Source: CAD feature listing. Evaluate the final solid. Frame: model axes, mm. A direction names the side the tool comes from. Coordinates: 2 decimals unless noted, no trailing zeros. Order: outer loops, then holes, each group sorted by start corner. A loop starts at its lowest first (then second) coordinate and runs counter-clockwise, first axis right, second up. Notation, with made-up numbers: (57, 57.25) - (97, 57.25) arc R24 cw to (97, 78.25) - close; hole circle Ø4 at (74.25, 22.25). An arc over 180 degrees is marked (long way). One line per question, with ' | ' between items.
from build123d import *

# Parameters (mm, degrees)
SKETCH1_R           = 60
BOSS_EXTRUDE1_DEPTH = 40
SKETCH2_R           = 30
BOSS_EXTRUDE2_DEPTH = 355
SKETCH3_W           = 35
SKETCH3_H           = 68.96676223
CUT_EXTRUDE1_DEPTH  = 45
SKETCH4_R           = 5
BOSS_EXTRUDE3_DEPTH = 35


with BuildPart() as part:
    # Sketch1 → Boss-Extrude1 (new body)
    with BuildSketch(Plane(origin=(0, 0, 0), x_dir=(0, 0, -1), z_dir=(1, 0, 0))):
        Circle(SKETCH1_R)
    extrude(amount=BOSS_EXTRUDE1_DEPTH)

    # Sketch2 → Boss-Extrude2 (add)
    with BuildSketch(Plane(origin=(40, 0, 0), x_dir=(0, 0, -1), z_dir=(1, 0, 0))):
        Circle(SKETCH2_R)
    extrude(amount=BOSS_EXTRUDE2_DEPTH)

    # Sketch3 → Cut-Extrude1 (cut)
    with BuildSketch(Plane(origin=(395, 0, 0), x_dir=(0, 0, -1), z_dir=(1, 0, 0))):
        Rectangle(SKETCH3_W, SKETCH3_H)
    extrude(amount=-CUT_EXTRUDE1_DEPTH, mode=Mode.SUBTRACT)

    # Sketch4 → Boss-Extrude3 (add)
    with BuildSketch(Plane.XY.offset(-17.5)):
        with Locations(Location((385, 0, 0), (0, 0, 180))):
            Circle(SKETCH4_R)
    extrude(amount=BOSS_EXTRUDE3_DEPTH)


solid = part.part
(1) Cut plane B-B (z = 0). Return the cut outline in (x, y), and give its area (3 significant figures).
Taken from the geometry:
outline: (0, -60) - (40, -60) - (40, -30) - (350, -30) - (350, 30) - (40, 30) - (40, 60) - (0, 60) - close; circle Ø10 at (385, 0) | area: 23,500 mm²
(2) Pin query (flat end, axial travel): P1, Ø12, axis at x = 104, z = 38, coming from the +Y side; P2, Ø13.5, axis at x = 369, y = 0.5, coming from the -Z side; P3, Ø5, axis at x = 327, y = 11.5, coming from the +Z side; P4, Ø6, axis at x = 115.5, z = 14, coming from the -Y side. Return the tip coordinate at first contact, or that it passes through.
Taken from the geometry:
P1: passes through | P2: stops at z = -30 | P3: stops at z = 28.62 | P4: stops at y = -27.91
(3) Material intervals for L1, parallel to X at y = -46.5, z = 34; L2, parallel to Y at x = 208.5, z = -2; L3, parallel to Z at x = 109, y = 13, sorted ascending. Write a range as from..to.
Taken from the geometry:
L1: x = 0..40 | L2: y = -29.93..29.93 | L3: z = -27.04..27.04
(4) Pull-direction query (Z, two-part tool) for faces 3 (the cylindrical face through (215.02, 1.32, 29.97)), 4 (the cylindrical face through (380.23, -1.5, -0.25)), 5 (the flat face through (395, 0, -22)); classes: pulls with the +Z half, pulls with the -Z half, needs draft (parallel to the pull), parting line crosses it, or undercut.
Taken from the geometry:
face 3: parting line crosses it | face 4: undercut | face 5: needs draft
(5) Cut plane D-D (z = -48). Return the cut outline in (x, y), and give its area (3 significant figures).
Taken from the geometry:
outline: (0, -36) - (40, -36) - (40, 36) - (0, 36) - close | area: 2,880 mm²
(6) Cut plane A-A (y = 0). Return the cut outline in (x, z).
Taken from the geometry:
outline: (0, -60) - (40, -60) - (40, -30) - (395, -30) - (395, -17.5) - (390, -17.5) - (390, 17.5) - (395, 17.5) - (395, 30) - (40, 30) - (40, 60) - (0, 60) - close; hole (350, -17.5) - (380, -17.5) - (380, 17.5) - (350, 17.5) - close
(7) Set-up query: faces 1 (the flat face through (0, 1, 1)), 2 (the flat face through (40, 28, -12)). Return all of +Z, -Z, +X, -X, +Y, -Y with unobstructed straight access to the full face (end or side cutting, diameter ignored); none if empty.
Taken from the geometry:
face 1: +Z, -Z, -X, +Y, -Y | face 2: +X
(8) Cut plane C-C (x = 385). Return the cut outline in (y, z).
Taken from the geometry:
outline: (-24.37, -17.5) arc R30 ccw to (24.37, -17.5) - (5, -17.5) - (5, 17.5) - (24.37, 17.5) arc R30 ccw to (-24.37, 17.5) - (-5, 17.5) - (-5, -17.5) - close
